The drawing under review shows one solid part. Ordinate dimensions are in mm from its lowest x, y, z. Give positions to 0.01 mm unless a question says otherwise; leave off trailing zeros. Order: outer loops, then holes, each group sorted by start corner. A loop starts at its lowest first (then second) coordinate and runs counter-clockwise, first axis right, second up. Notation, with made-up numbers: M 4,-17 L 37,-17 A22 cw 37,3 Z; hole C 52.5,50 d11. An arc over 180 degrees is marked long. Put each result on its own line as item: value. Start each with the question number.
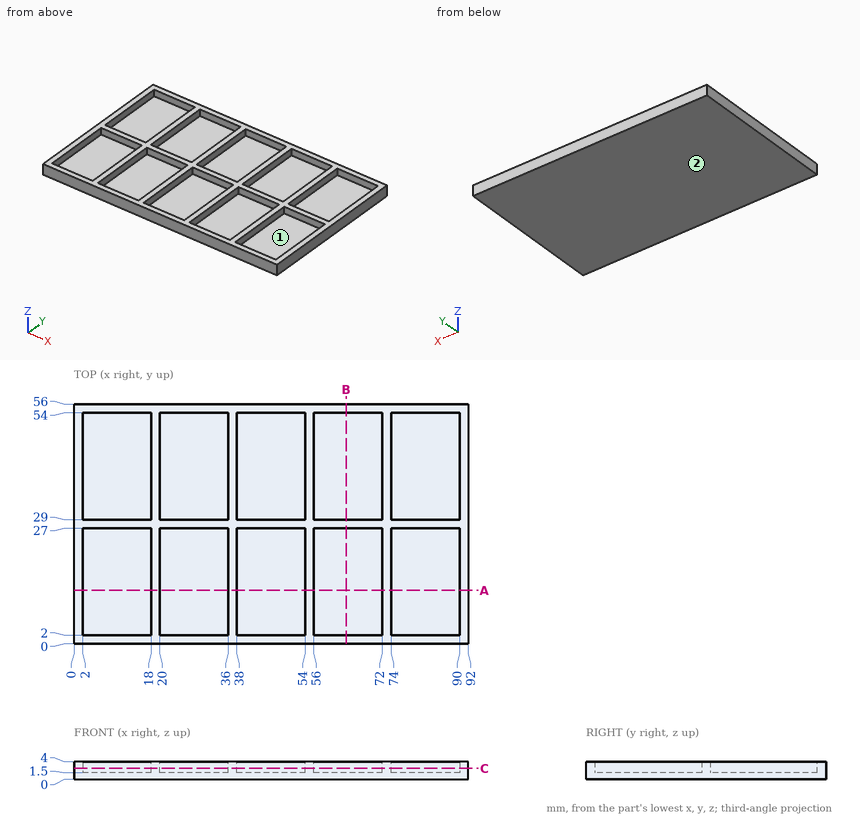
1. Consider section B-B on x = 63.5. Give the boundary of the cut face in (y, z), then the cut area to 3 significant figures.
2. Insertion check: pin 1 (5 mm diameter, centred on x = 6.5, y = 40.5, fed in from +Z). The pin has a flat end and moves straight along its axis. Give the tip position at first contact, or say it passes through.
3. Consider section A-A on y = 12.5. Give the boundary of the cut face in (x, z), then the cut area to 3 significant figures.
4. The part is to be moulded in two halves that separate along X. For the marked faces 1 and 2, say which applies: +X half, -X half, draft (parallel to the pull), parting line (faces both ways), or undercut.
5. Consider section C-C on z = 2.5. Give the number of separate pieces and of enclosed holes in the cut face, then the cut area to 3 significant figures.
6. To check wall thickness, follow probe 1 along X at (y, z) = (50.5, 2.9); probe 2 along Y at (x, z) = (78, 2.6); probe 3 along Z at (x, y) = (4, 26). State the ranges of each line that lie inside material, in increasing order.
Returned:
1. outline: M 0,0 L 56,0 L 56,4 L 54,4 L 54,1.5 L 29,1.5 L 29,4 L 27,4 L 27,1.5 L 2,1.5 L 2,4 L 0,4 Z
1. area: 99.0 mm2
2. pin 1: stops at z = 1.5
3. outline: M 0,0 L 92,0 L 92,4 L 90,4 L 90,1.5 L 74,1.5 L 74,4 L 72,4 L 72,1.5 L 56,1.5 L 56,4 L 54,4 L 54,1.5 L 38,1.5 L 38,4 L 36,4 L 36,1.5 L 20,1.5 L 20,4 L 18,4 L 18,1.5 L 2,1.5 L 2,4 L 0,4 Z
3. area: 168 mm2
4. face 1: undercut
4. face 2: draft
5. separate pieces: 1
5. enclosed holes: 10
5. area: 1,150 mm2
6. probe 1: x = 0 to 2, 18 to 20, 36 to 38, 54 to 56, 72 to 74, 90 to 92
6. probe 2: y = 0 to 2, 27 to 29, 54 to 56
6. probe 3: z = 0 to 1.5
